Here's how the part is built. I have some questions about the finished solid (model axes, mm). Face numbers are marked on the shaded views. Coordinates: 2 decimals unless noted, no trailing zeros. Order: outer loops, then holes, each group sorted by start corner. A loop starts at its lowest first (then second) coordinate and runs counter-clockwise, first axis right, second up.
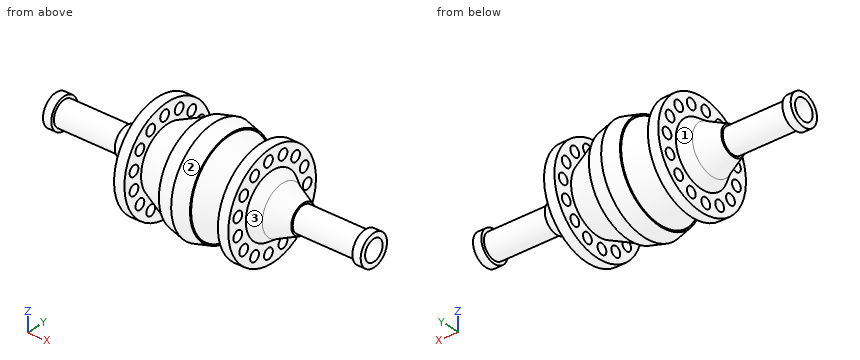
```python
from build123d import *

# Parameters (mm, degrees)
SKETCH1_R                     = 25
BOSS_EXTRUDE1_DEPTH           = 7.5
BOSS_EXTRUDE1_TAPER           = 14
BOSS_EXTRUDE1_OTHER_WAY_DEPTH = 7.5
BOSS_EXTRUDE1_OTHER_WAY_TAPER = 14
SKETCH2_R                     = 22.5
BOSS_EXTRUDE2_DEPTH           = 15
BOSS_EXTRUDE2_TAPER           = 25
SKETCH3_R                     = 22.5
BOSS_EXTRUDE3_DEPTH           = 15
BOSS_EXTRUDE3_TAPER           = 25
SKETCH4_R                     = 25
BOSS_EXTRUDE4_DEPTH           = 5
BOSS_EXTRUDE5_START           = 5
SKETCH5_R                     = 25
BOSS_EXTRUDE5_DEPTH           = 5
SKETCH6_R                     = 2.5
CUT_EXTRUDE1_DEPTH            = 5
CUT_EXTRUDE2_START            = -50
SKETCH6_2_R                   = 2.5
CUT_EXTRUDE2_DEPTH            = 5
SKETCH7_R                     = 15
BOSS_EXTRUDE6_DEPTH           = 5
BOSS_EXTRUDE6_TAPER           = 35
SKETCH8_R                     = 11.498962309
BOSS_EXTRUDE7_DEPTH           = 10
BOSS_EXTRUDE7_TAPER           = 25
SKETCH10_R                    = 6
BOSS_EXTRUDE8_DEPTH           = 30
SKETCH11_R                    = 7.5
BOSS_EXTRUDE10_DEPTH          = 4
SKETCH14_R                    = 15
BOSS_EXTRUDE11_DEPTH          = 5
BOSS_EXTRUDE11_TAPER          = 35
SKETCH16_R                    = 11.509262746
BOSS_EXTRUDE12_DEPTH          = 10
BOSS_EXTRUDE12_TAPER          = 25
BOSS_EXTRUDE13_START          = 30
SKETCH17_R                    = 6
BOSS_EXTRUDE13_DEPTH          = 30
BOSS_EXTRUDE14_START          = 4
SKETCH18_R                    = 7.5
BOSS_EXTRUDE14_DEPTH          = 4
CUT_EXTRUDE3_START            = -153
SKETCH20_R                    = 5
CUT_EXTRUDE3_DEPTH            = 153


with BuildPart() as part:
    # Sketch1 → Boss-Extrude1 (new body)
    with BuildSketch(Plane(origin=(0, 0, 0), x_dir=(0, 0, -1), z_dir=(1, 0, 0))):
        Circle(SKETCH1_R)
    extrude(amount=BOSS_EXTRUDE1_DEPTH, taper=BOSS_EXTRUDE1_TAPER)

    # Sketch1 → Boss-Extrude1 other way (add)
    with BuildSketch(Plane(origin=(0, 0, 0), x_dir=(0, 0, -1), z_dir=(1, 0, 0))):
        Circle(SKETCH1_R)
    extrude(amount=-BOSS_EXTRUDE1_OTHER_WAY_DEPTH, taper=BOSS_EXTRUDE1_OTHER_WAY_TAPER)

    # Sketch2 → Boss-Extrude2 (add)
    with BuildSketch(Plane.ZY.offset(7.5)):
        Circle(SKETCH2_R)
    extrude(amount=BOSS_EXTRUDE2_DEPTH, taper=BOSS_EXTRUDE2_TAPER)

    # Sketch3 → Boss-Extrude3 (add)
    with BuildSketch(Plane(origin=(7.5, 0, 0), x_dir=(0, 0, -1), z_dir=(1, 0, 0))):
        Circle(SKETCH3_R)
    extrude(amount=BOSS_EXTRUDE3_DEPTH, taper=BOSS_EXTRUDE3_TAPER)

    # Sketch4 → Boss-Extrude4 (add)
    with BuildSketch(Plane(origin=(22.5, 0, 0), x_dir=(0, 0, -1), z_dir=(1, 0, 0))):
        Circle(SKETCH4_R)
    extrude(amount=BOSS_EXTRUDE4_DEPTH)

    # Sketch5 → Boss-Extrude5 (add)
    with BuildSketch(Plane.ZY.offset(22.5).offset(BOSS_EXTRUDE5_START)):
        with Locations(Location((0, 0, 0), (0, 0, 180))):
            Circle(SKETCH5_R)
    extrude(amount=-BOSS_EXTRUDE5_DEPTH)

    # Sketch6 → Cut-Extrude1 (cut)
    with BuildSketch(Plane.ZY.offset(27.5)):
        with Locations((0, 20)):
            Circle(SKETCH6_R)
        with Locations((8.134732862, 18.270909153)):
            Circle(SKETCH6_R)
        with Locations((14.86289651, 13.382612127)):
            Circle(SKETCH6_R)
        with Locations((19.021130326, 6.180339888)):
            Circle(SKETCH6_R)
        with Locations((19.890437907, -2.090569265)):
            Circle(SKETCH6_R)
        with Locations((17.320508076, -10)):
            Circle(SKETCH6_R)
        with Locations((11.755705046, -16.180339887)):
            Circle(SKETCH6_R)
        with Locations((4.158233816, -19.562952015)):
            Circle(SKETCH6_R)
        with Locations((-4.158233816, -19.562952015)):
            Circle(SKETCH6_R)
        with Locations((-11.755705046, -16.180339888)):
            Circle(SKETCH6_R)
        with Locations((-17.320508076, -10)):
            Circle(SKETCH6_R)
        with Locations((-19.890437907, -2.090569265)):
            Circle(SKETCH6_R)
        with Locations((-19.021130326, 6.180339887)):
            Circle(SKETCH6_R)
        with Locations((-14.86289651, 13.382612127)):
            Circle(SKETCH6_R)
        with Locations((-8.134732862, 18.270909153)):
            Circle(SKETCH6_R)
    extrude(amount=-CUT_EXTRUDE1_DEPTH, mode=Mode.SUBTRACT)

    # Sketch6<2> → Cut-Extrude2 (cut)
    with BuildSketch(Plane.ZY.offset(27.5).offset(CUT_EXTRUDE2_START)):
        with Locations((0, 20)):
            Circle(SKETCH6_2_R)
        with Locations((8.134732862, 18.270909153)):
            Circle(SKETCH6_2_R)
        with Locations((14.86289651, 13.382612127)):
            Circle(SKETCH6_2_R)
        with Locations((19.021130326, 6.180339888)):
            Circle(SKETCH6_2_R)
        with Locations((19.890437907, -2.090569265)):
            Circle(SKETCH6_2_R)
        with Locations((17.320508076, -10)):
            Circle(SKETCH6_2_R)
        with Locations((11.755705046, -16.180339887)):
            Circle(SKETCH6_2_R)
        with Locations((4.158233816, -19.562952015)):
            Circle(SKETCH6_2_R)
        with Locations((-4.158233816, -19.562952015)):
            Circle(SKETCH6_2_R)
        with Locations((-11.755705046, -16.180339888)):
            Circle(SKETCH6_2_R)
        with Locations((-17.320508076, -10)):
            Circle(SKETCH6_2_R)
        with Locations((-19.890437907, -2.090569265)):
            Circle(SKETCH6_2_R)
        with Locations((-19.021130326, 6.180339887)):
            Circle(SKETCH6_2_R)
        with Locations((-14.86289651, 13.382612127)):
            Circle(SKETCH6_2_R)
        with Locations((-8.134732862, 18.270909153)):
            Circle(SKETCH6_2_R)
    extrude(amount=-CUT_EXTRUDE2_DEPTH, mode=Mode.SUBTRACT)

    # Sketch7 → Boss-Extrude6 (add)
    with BuildSketch(Plane.ZY.offset(27.5)):
        Circle(SKETCH7_R)
    extrude(amount=BOSS_EXTRUDE6_DEPTH, taper=BOSS_EXTRUDE6_TAPER)

    # Sketch8 → Boss-Extrude7 (add)
    with BuildSketch(Plane.ZY.offset(32.5)):
        Circle(SKETCH8_R)
    extrude(amount=BOSS_EXTRUDE7_DEPTH, taper=BOSS_EXTRUDE7_TAPER)

    # Sketch10 → Boss-Extrude8 (add)
    with BuildSketch(Plane.ZY.offset(42.5)):
        Circle(SKETCH10_R)
    extrude(amount=BOSS_EXTRUDE8_DEPTH)

    # Sketch11 → Boss-Extrude10 (add)
    with BuildSketch(Plane.ZY.offset(72.5)):
        Circle(SKETCH11_R)
    extrude(amount=BOSS_EXTRUDE10_DEPTH)

    # Sketch14 → Boss-Extrude11 (add)
    with BuildSketch(Plane(origin=(27.5, 0, 0), x_dir=(0, 0, -1), z_dir=(1, 0, 0))):
        Circle(SKETCH14_R)
    extrude(amount=BOSS_EXTRUDE11_DEPTH, taper=BOSS_EXTRUDE11_TAPER)

    # Sketch16 → Boss-Extrude12 (add)
    with BuildSketch(Plane(origin=(32.5, 0, 0), x_dir=(0, 0, -1), z_dir=(1, 0, 0))):
        Circle(SKETCH16_R)
    extrude(amount=BOSS_EXTRUDE12_DEPTH, taper=BOSS_EXTRUDE12_TAPER)

    # Sketch17 → Boss-Extrude13 (add)
    with BuildSketch(Plane(origin=(42.5, 0, 0), x_dir=(0, 0, -1), z_dir=(1, 0, 0)).offset(BOSS_EXTRUDE13_START)):
        with Locations(Location((0, 0, 0), (0, 0, 180))):
            Circle(SKETCH17_R)
    extrude(amount=-BOSS_EXTRUDE13_DEPTH)

    # Sketch18 → Boss-Extrude14 (add)
    with BuildSketch(Plane(origin=(72.5, 0, 0), x_dir=(0, 0, -1), z_dir=(1, 0, 0)).offset(BOSS_EXTRUDE14_START)):
        with Locations(Location((0, 0, 0), (0, 0, 180))):
            Circle(SKETCH18_R)
    extrude(amount=-BOSS_EXTRUDE14_DEPTH)

    # Sketch20 → Cut-Extrude3 (cut)
    with BuildSketch(Plane.ZY.offset(76.5).offset(CUT_EXTRUDE3_START)):
        Circle(SKETCH20_R)
    cut_extrude3 = extrude(amount=CUT_EXTRUDE3_DEPTH, mode=Mode.SUBTRACT)

    # Mirror1: Cut-Extrude3 across plane
    add(cut_extrude3.mirror(Plane(origin=(0, 0, 0), x_dir=(0, 0, 1), z_dir=(1, 0, 0))), mode=Mode.SUBTRACT)


solid = part.part
```
Q1. If we section it at B-B on z = 0: Give the number of separate pieces and of enclosed holes in the cut face, then the cut area to 3 significant figures.
Q2. If we section it at A-A on x = 58.5: Write out the boundary of the cut face in (y, z).
Q3. If we section it at D-D on x = -21: Write out the boundary of the cut face in (y, z).
Q4. I need wall thicknesses on L1, parallel to X at y = 22, z = -5; L2, parallel to X at y = -3, z = 5.5; L3, parallel to Y at x = -3, z = -4.5. Which ranges of each line are inside material? Lowest first, please.
Q5. We'd pull the mould along X, two halves only. Please class the marked faces 1, 2 and 3: pulls with the +X half, pulls with the -X half, needs draft (parallel to the pull), parting line crosses it, or undercut.
Q6. Will these pins go through, and if not, where does the flat tip stop? pin 1 (5 mm diameter, centred on x = -55, y = 10, fed in from +Z); pin 2 (3 mm diameter, centred on y = 18.27, z = -8.13, fed in from -X); pin 3 (1 mm diameter, centred on x = 3, z = 7.5, fed in from +Y); pin 4 (10 mm diameter, centred on y = 6.5, z = 19.5, fed in from -X).
Reply:
1. separate pieces: 4
1. enclosed holes: 0
1. area: 2,250 mm2
2. outline: circle Ø12 at (0, 0); hole circle Ø10 at (0, 0)
3. outline: circle Ø32.41 at (0, 0); hole circle Ø10 at (0, 0)
4. L1: x = -27.5 to -22.5, -7.5 to 7.5, 22.5 to 27.5
4. L2: x = -76.5 to -72.5, -42.5 to 42.5, 72.5 to 76.5
4. L3: y = -23.83 to -2.18, 2.18 to 23.83
5. face 1: pulls with the -X half
5. face 2: undercut
5. face 3: pulls with the +X half
6. pin 1: passes through
6. pin 2: stops at x = -16.08
6. pin 3: stops at y = 23.27
6. pin 4: stops at x = -27.5
